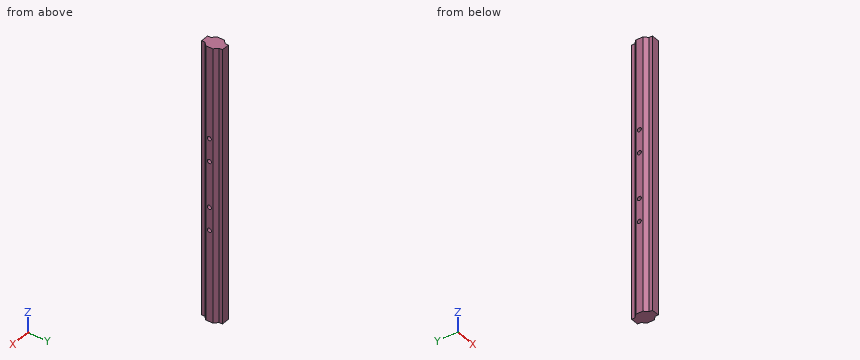
```python
from build123d import *

# Parameters (mm, degrees)
BOSS_EXTRUDE1_DEPTH = 200
SKETCH2_R           = 1.5
CUT_EXTRUDE1_DEPTH  = 20


with BuildPart() as part:
    # Sketch1 → Boss-Extrude1 (new body)
    with BuildSketch(Plane.XY.offset(116.106580091)):
        Polygon((-39.550290087, 5.294235639), (-36.889629915, 7.954895811), (-36.889629915, 10.362002592), (-31.010950259, 10.362002592), (-31.010950259, 7.954895811), (-28.350290087, 5.294235639), (-28.350290087, 0.029769545), (-31.010950259, -2.630890626), (-31.010950259, -5.037997408), (-36.889629915, -5.037997408), (-36.889629915, -2.630890626), (-39.550290087, 0.029769545), align=None)
    extrude(amount=BOSS_EXTRUDE1_DEPTH)

    # Sketch2 → Cut-Extrude1 (cut)
    with BuildSketch(Plane(origin=(-28.350290087, 0, 0), x_dir=(0, 0, -1), z_dir=(1, 0, 0))):
        with Locations((-232.806580091, 2.662002592)):
            Circle(SKETCH2_R)
        with Locations((-249.506580091, 2.662002592)):
            Circle(SKETCH2_R)
        with Locations((-199.406580091, 2.662002592)):
            Circle(SKETCH2_R)
        with Locations((-182.706580091, 2.662002592)):
            Circle(SKETCH2_R)
    extrude(amount=-CUT_EXTRUDE1_DEPTH, mode=Mode.SUBTRACT)


solid = part.part
```
Can you work these out from the model? Positions are in its coordinate system, mm. Round coordinates to 2 decimals unless told otherwise and drop trailing zeros. Loops run counter-clockwise (first coordinate to the right, second up) from the corner with the lowest first, then second, coordinate; pieces in that order, holes last.
Item 1: Will these pins go through, and if not, where does the flat tip stop? pin 1 Ø2.5 at (y, z) = (-3.5, 227) entering from -X; pin 2 Ø2.5 at (y, z) = (-3.5, 195) entering from +X; pin 3 Ø1.9 at (y, z) = (9, 225) entering from -X.
Item 2: Suppose I cut it at A-A, the plane z = 255.5. Write out the boundary of the cut face in (x, y), then the cut area to 3 significant figures.
Item 3: Please list where these lines run through material, in increasing order: L1, parallel to Z at x = -33, y = 2; L2, parallel to X at y = -3.75, z = 191; L3, parallel to Y at x = -36, z = 233.
Reported:
1. pin 1: stops at x = -37.27
1. pin 2: stops at x = -30.63
1. pin 3: stops at x = -36.89
2. outline: (-39.55, 0.03) - (-36.89, -2.63) - (-36.89, -5.04) - (-31.01, -5.04) - (-31.01, -2.63) - (-28.35, 0.03) - (-28.35, 5.29) - (-31.01, 7.95) - (-31.01, 10.36) - (-36.89, 10.36) - (-36.89, 7.95) - (-39.55, 5.29) - close
2. area: 133 mm2
3. L1: z = 116.11 to 181.36, 184.05 to 198.06, 200.75 to 231.46, 234.15 to 248.16, 250.85 to 316.11
3. L2: x = -36.89 to -31.01
3. L3: y = -5.04 to 1.17, 4.15 to 10.36
